```python
from build123d import *

# Parameters (mm, degrees)
F0_W     = 500
F0_H     = 200
F0_R     = 14
F0_R_2   = 17
F0_R_3   = 26.5
F1_DEPTH = 75
F2_T     = -8
F3_R     = 5


with BuildPart() as f1:
    # F0 (on Front) → F1 (new body, symmetric)
    with BuildSketch(Plane.XZ):
        Rectangle(F0_W, F0_H)
        with Locations((-210, 0)):
            Circle(F0_R, mode=Mode.SUBTRACT)
        with Locations((-140, 0)):
            Circle(F0_R, mode=Mode.SUBTRACT)
        with Locations((-70, 0)):
            Circle(F0_R, mode=Mode.SUBTRACT)
        Circle(F0_R_2, mode=Mode.SUBTRACT)
        with Locations((80, 0)):
            Circle(F0_R_3, mode=Mode.SUBTRACT)
        with Locations((-210, 0)):
            Circle(F0_R)
        with Locations((-140, 0)):
            Circle(F0_R)
        with Locations((-70, 0)):
            Circle(F0_R)
        Circle(F0_R_2)
        with Locations((80, 0)):
            Circle(F0_R_3)
    extrude(amount=F1_DEPTH, both=True)

    # F2
    f2_openings = [f1.faces().sort_by_distance(p)[0] for p in [
        (250, 0, 0),
        (-250, 0, 0),
    ]]
    offset(amount=F2_T, openings=f2_openings)

    # F3
    f3_edges = [f1.edges().sort_by_distance(p)[0] for p in [
        (0, 75, 100),
        (0, -75, -100),
        (250, -75, 0),
        (0, -75, 100),
        (-250, -75, 0),
        (250, 0, 100),
        (-250, 0, 100),
        (0, 75, -100),
        (250, 0, -100),
        (-250, 0, -100),
    ]]
    fillet(f3_edges, radius=F3_R)


solid = f1.part
```
Verification items for the finished model (mm, model axes). A direction names the side the tool comes from. Round coordinates to 2 decimals unless told otherwise and drop trailing zeros. Order: outer loops, then holes, each group sorted by start corner. A loop starts at its lowest first (then second) coordinate and runs counter-clockwise, first axis right, second up. Notation, with made-up numbers: (71.25, 51) -> (114.25, 51) arc R20 ccw to (114.25, 57) -> close; hole circle Ø6 at (83, 61). An arc over 180 degrees is marked (long way). Put each result on its own line as item: value. Start each with the question number.
(1) Section check C-C (x = 44). Enter the section's corners in (y, z).
(2) Tool access check on faces 4 (the face through (250, -68, 0)), 5 (the face through (-3, -67, 1)). Record the directions out of +Z, -Z, +X, -X, +Y, -Y that give a thin tool (end or side, any length) a straight path to the whole face; none if there is none.
(3) Material ranges on line 1 along Z through (x, y) = (-23, 44); line 2 along Y through (x, z) = (180.5, -16.5), recorded low to high.
(4) Section check A-A (z = 35.5). Enter the section's corners in (x, y), then the cut area to 3 significant figures.
(5) Section check B-B (y = -30). Enter the section's corners in (x, z).
(6) Draft check along Y on faces 1 (the face through (-3, -1, 100)), 2 (the face through (-3, -1, 92)), 3 (the face through (-3, 75, 1)). Enter one of: +Y half, -Y half, draft (parallel to the pull), parting line (faces both ways), or undercut.
Completed:
1. outline: (-75, -95) arc R5 ccw to (-70, -100) -> (70, -100) arc R5 ccw to (75, -95) -> (75, 95) arc R5 ccw to (70, 100) -> (-70, 100) arc R5 ccw to (-75, 95) -> close; hole (-67, -92) -> (67, -92) -> (67, 92) -> (-67, 92) -> close
2. face 4: +Z, -Z, +X, +Y, -Y
2. face 5: +X, -X
3. line 1: z = -100 to -92, 92 to 100
3. line 2: y = -75 to -67, 67 to 75
4. outline: (-250, -70) arc R5 ccw to (-245, -75) -> (245, -75) arc R5 ccw to (250, -70) -> (250, -67) -> (-250, -67) -> close; (-250, 67) -> (250, 67) -> (250, 75) -> (-250, 75) -> close
4. area: 7,990 mm2
5. outline: (-250, -95) arc R5 ccw to (-245, -100) -> (245, -100) arc R5 ccw to (250, -95) -> (250, -92) -> (-250, -92) -> close; (-250, 92) -> (250, 92) -> (250, 95) arc R5 ccw to (245, 100) -> (-245, 100) arc R5 ccw to (-250, 95) -> close
6. face 1: draft
6. face 2: undercut
6. face 3: +Y half
